```python
from build123d import *

# Parameters (mm, degrees)
SZKIC1_W                = 130
SZKIC1_H                = 20
ODGI_CIE_BAZOWE1_DEPTH  = 1.5
OTW_R_POD_RUB_M51_D     = 5.5
OTW_R_POD_RUB_M51_DEPTH = 10
OTW_R_POD_RUB_M51_TIP   = 1.652366702
ZAOKR_GLENIE1_R         = 3


# Sheet-metal steps are written as plain solids
with BuildPart() as part:
    # Szkic1 → Odgięcie bazowe1 (new body)
    with BuildSketch(Plane(origin=(0, 0, 0), x_dir=(0, 0, -1), z_dir=(1, 0, 0))):
        Rectangle(SZKIC1_W, SZKIC1_H)
    extrude(amount=-ODGI_CIE_BAZOWE1_DEPTH)

    # Otwór pod śrubę M51
    with Locations(Plane(origin=(0, 0, 0), x_dir=(0, 0, -1), z_dir=(1, 0, 0))):
        with Locations((-10, 0), (50, 0)):
            Hole(OTW_R_POD_RUB_M51_D / 2, depth=OTW_R_POD_RUB_M51_DEPTH)
            with Locations((0, 0, -(OTW_R_POD_RUB_M51_DEPTH + OTW_R_POD_RUB_M51_TIP / 2))):  # 118° drill point
                Cone(0, OTW_R_POD_RUB_M51_D / 2, OTW_R_POD_RUB_M51_TIP, mode=Mode.SUBTRACT)

    # Zaokrąglenie1
    zaokr_glenie1_edges = [part.edges().sort_by_distance(p)[0] for p in [
        (-0.75, -10, -65),
        (-0.75, -10, 65),
        (-0.75, 10, 65),
        (-0.75, 10, -65),
    ]]
    fillet(zaokr_glenie1_edges, radius=ZAOKR_GLENIE1_R)


solid = part.part
```
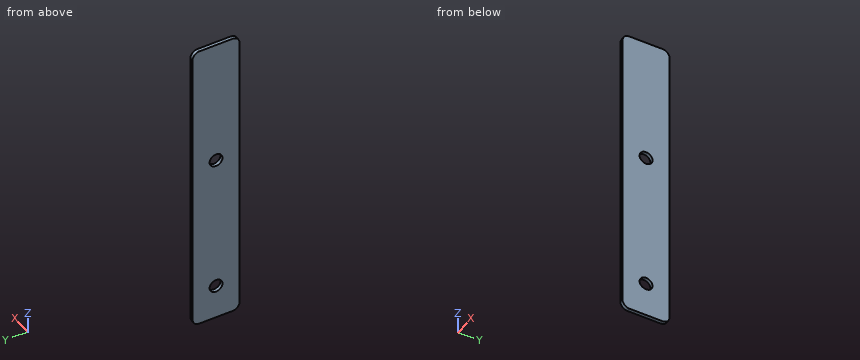
Verification items for the finished model (mm, model axes). Round coordinates to 2 decimals unless told otherwise and drop trailing zeros. Write each loop counter-clockwise with the first axis right and the second up, starting at its lowest first coordinate (ties: lowest second). Pieces come first, ordered by that corner, then holes.
1. Section check B-B on y = 0. Enter the section's corners in (x, z).
2. Section check A-A on z = -50. Enter the section's corners in (x, y), plus the area to 4 significant figures.
3. Scan lines: L1, parallel to Y at x = -0.4, z = 10; L2, parallel to Z at x = -1.25, y = -2; L3, parallel to Z at x = -1.3, y = 8.25. Record each from-to range of solid material in increasing order.
4. Section check C-C on x = -0.95. Enter the section's corners in (y, z), plus the area to 3 significant figures.
Answer:
1. outline: (-1.5, -65) - (0, -65) - (0, -52.75) - (-1.5, -52.75) - close; (-1.5, -47.25) - (0, -47.25) - (0, 7.25) - (-1.5, 7.25) - close; (-1.5, 12.75) - (0, 12.75) - (0, 65) - (-1.5, 65) - close
2. outline: (-1.5, -10) - (0, -10) - (0, -2.75) - (-1.5, -2.75) - close; (-1.5, 2.75) - (0, 2.75) - (0, 10) - (-1.5, 10) - close
2. area: 21.75 mm2
3. L1: y = -10 to -2.75, 2.75 to 10
3. L2: z = -65 to -51.89, -48.11 to 8.11, 11.89 to 65
3. L3: z = -64.73 to 64.73
4. outline: (-10, -62) arc R3 ccw to (-7, -65) - (7, -65) arc R3 ccw to (10, -62) - (10, 62) arc R3 ccw to (7, 65) - (-7, 65) arc R3 ccw to (-10, 62) - close; hole circle Ø5.5 at (0, -50); hole circle Ø5.5 at (0, 10)
4. area: 2,540 mm2
